Part print with two shaded views. Sizes in mm from the minimum x, y, z corner. A direction names the side the tool comes from. Coordinates: 2 decimals unless noted, no trailing zeros. Write each loop counter-clockwise with the first axis right and the second up, starting at its lowest first coordinate (ties: lowest second). Pieces come first, ordered by that corner, then holes.
Q1. Drill centre lines: probe 1 along Y at (x, z) = (0.5, 8.25); probe 2 along Z at (x, y) = (2.5, 8); probe 3 along Z at (x, y) = (7, 10). Where is each one in solid material? Low to high.
Q2. Band-saw the part on D-D, the plane y = 4. Write the cut outline in (x, z).
Q3. Pin check, flat tips, straight feed: P1, Ø4, axis at y = 4, z = 2, coming from the +X side; P2, Ø3, axis at x = 9, y = 2, coming from the +Z side; P3, Ø2, axis at x = 9, z = 10, coming from the -Y side; P4, Ø1.5, axis at x = 1.5, y = 2.5, coming from the -Z side. Stop position of each tip, or through.
Q4. Band-saw the part on C-C, the plane y = 9.5. Write the cut outline in (x, z), plus the area to 3 significant figures.
Q5. Which spindle directions (+Z, -Z, +X, -X, +Y, -Y) get a long thin tool onto all of the face, cutting with end or side? Do the marked faces 1 and 2. Say none if no direction does.
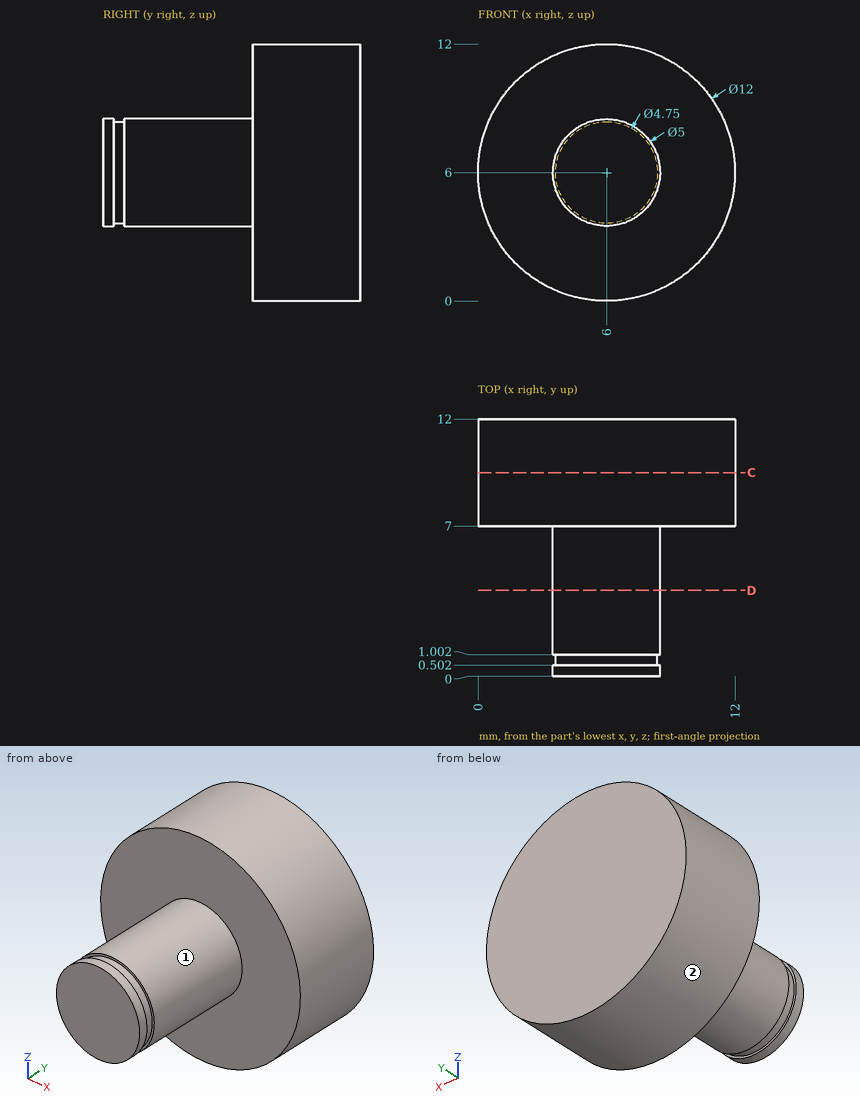
Answer sheet:
1. probe 1: y = 7 to 12
1. probe 2: z = 1.13 to 10.87
1. probe 3: z = 0.08 to 11.92
2. outline: circle Ø5 at (6, 6)
3. P1: stops at x = 7.5
3. P2: stops at z = 8
3. P3: stops at y = 7
3. P4: passes through
4. outline: circle Ø12 at (6, 6)
4. area: 113 mm2
5. face 1: -Y
5. face 2: +Y, -Y
